CAD build for the part. Positions are in the model's coordinates, mm. Coordinates: 2 decimals unless noted, no trailing zeros. Write each loop counter-clockwise with the first axis right and the second up, starting at its lowest first coordinate (ties: lowest second). Pieces come first, ordered by that corner, then holes.
```python
from build123d import *

# Parameters (mm, degrees)
F1_DEPTH = 5.08
F2_D     = 21
F3_D     = 6.35
F4_D     = 6.35
F5_D     = 6.35


with BuildPart() as f1:
    # F0 (on Top) → F1 (new body)
    with BuildSketch(Plane.XY):
        with BuildLine():
            Line((26.5037064396, -9.4034548087), (4.9663911618, 27.6804330928))
            ThreePointArc((4.9663911618, 27.6804330928), (-0.0783700027, 30.5758122309), (-5.1082224721, 27.6546104755))
            Line((-5.1082224721, 27.6546104755), (-26.455153827, -9.5391956352))
            ThreePointArc((-26.455153827, -9.5391956352), (-26.440245132, -15.3557765287), (-21.3954839675, -18.2511556668))
            Line((-21.3954839675, -18.2511556668), (21.4887626653, -18.1412374576))
            ThreePointArc((21.4887626653, -18.1412374576), (26.5186151347, -15.2200357022), (26.5037064396, -9.4034548087))
        make_face()
    extrude(amount=F1_DEPTH)

    # F2 (through all)
    with Locations(Plane(origin=(0, 0, 0), x_dir=(1, 0, 0), z_dir=(0, 0, -1))):
        with Locations((0, 0)):
            Hole(F2_D / 2)

    # F3 (through all)
    with Locations(Plane(origin=(0, 0, 0), x_dir=(1, 0, 0), z_dir=(0, 0, -1))):
        with Locations((-21.4103926626, 12.4345747733)):
            Hole(F3_D / 2)

    # F4 (through all)
    with Locations(Plane(origin=(0, 0, 0), x_dir=(1, 0, 0), z_dir=(0, 0, -1))):
        with Locations((21.4738539702, 12.3246565641)):
            Hole(F4_D / 2)

    # F5 (through all)
    with Locations(Plane(origin=(0, 0, 0), x_dir=(1, 0, 0), z_dir=(0, 0, -1))):
        with Locations((-0.0634613077, -24.7592313374)):
            Hole(F5_D / 2)


solid = f1.part
```
Item 1: Saw through at B-B, the plane y = -14. Write the cut outline in (x, z).
Item 2: Saw through at A-A, the plane x = 7.5. Write the cut outline in (y, z), and give its area (3 significant figures).
Item 3: Flat gauge pins, fed straight in: pin 1 Ø12 at (x, y) = (21.5, 22.5) entering from -Z; pin 2 Ø3 at (x, z) = (-21.5, 2.5) entering from +Y; pin 3 Ø2 at (y, z) = (10, 1) entering from -X; pin 4 Ø2 at (x, z) = (10.5, 2.5) entering from +Y. Where does each tip first touch, or does it go through?
Item 4: Saw through at D-D, the plane y = 0. Write the cut outline in (x, z), and give its area (3 significant figures).
Item 5: Saw through at C-C, the plane x = 0. Write the cut outline in (y, z), and give its area (3 significant figures).
Item 6: Two-plate mould, pull along X, no slides. Class faces 1 (the cylindrical face through (0.007, 30.575, 2.504)), 2 (the cylindrical face through (-24.343, -11.219, 2.576)), 3 (the cylindrical face through (-10, -3.2, 2.6)), 4 (the flat face through (-6, -10, 5.08)): +X half, -X half, draft (parallel to the pull), parting line (faces both ways), or undercut.
Item 7: Wall check: line 1 along Y through (x, z) = (0.5, 3.4); line 2 along Y through (x, z) = (0, 2.5); line 3 along X through (y, z) = (-6.5, 1.15). Give the ranges that are in metal, low to high.
Working result:
1. outline: (-27.01, 0) - (-24.17, 0) - (-24.17, 5.08) - (-27.01, 5.08) - close; (-18.65, 0) - (18.78, 0) - (18.78, 5.08) - (-18.65, 5.08) - close; (24.17, 0) - (27.04, 0) - (27.04, 5.08) - (24.17, 5.08) - close
2. outline: (-18.18, 0) - (-7.35, 0) - (-7.35, 5.08) - (-18.18, 5.08) - close; (7.35, 0) - (23.32, 0) - (23.32, 5.08) - (7.35, 5.08) - close
2. area: 136 mm2
3. pin 1: passes through
3. pin 2: stops at y = 1.71
3. pin 3: stops at x = -15.81
3. pin 4: stops at y = 19.87
4. outline: (-20.98, 0) - (-10.5, 0) - (-10.5, 5.08) - (-20.98, 5.08) - close; (10.5, 0) - (21.04, 0) - (21.04, 5.08) - (10.5, 5.08) - close
4. area: 107 mm2
5. outline: (-18.2, 0) - (-10.5, 0) - (-10.5, 5.08) - (-18.2, 5.08) - close; (10.5, 0) - (21.58, 0) - (21.58, 5.08) - (10.5, 5.08) - close; (27.93, 0) - (30.58, 0) - (30.58, 5.08) - (27.93, 5.08) - close
5. area: 109 mm2
6. face 1: parting line
6. face 2: undercut
6. face 3: undercut
6. face 4: draft
7. line 1: y = -18.2 to -10.49, 10.49 to 21.63, 27.88 to 30.55
7. line 2: y = -18.2 to -10.5, 10.5 to 21.58, 27.93 to 30.58
7. line 3: x = -24.71 to -8.25, 8.25 to 24.82
